Source: CAD feature listing. Evaluate the final solid. Frame: model axes, mm. Give positions to 0.01 mm unless a question says otherwise; leave off trailing zeros. Write each loop counter-clockwise with the first axis right and the second up, starting at its lowest first coordinate (ties: lowest second). Pieces come first, ordered by that corner, then holes. Notation, with made-up numbers: (73, 13.5) -> (112, 13.5) arc R15 cw to (112, 39.5) -> close; hole circle Ø2 at (55, -31). An arc over 180 degrees is marked (long way). Write item = value, one per line.
from build123d import *

# Parameters (mm, degrees)
SKETCH_1_W          = 148.2
SKETCH_1_H          = 100
SKETCH_1_W_2        = 144.2
SKETCH_1_H_2        = 96
EXTRUDE_1_DEPTH     = 4
SKETCH_2_R          = 0.4
CUT_EXTRUDE_1_DEPTH = 125.526342595
SKETCH_3_R          = 0.4
CUT_EXTRUDE_2_DEPTH = 157.458428984


with BuildPart() as part:
    # 草图1 → 凸台-拉伸1 (new body)
    with BuildSketch(Plane(origin=(0, 0, 0), x_dir=(1, 0, 0), z_dir=(0, 1, 0))):
        Rectangle(SKETCH_1_W, SKETCH_1_H)
        Rectangle(SKETCH_1_W_2, SKETCH_1_H_2, mode=Mode.SUBTRACT)
    extrude(amount=EXTRUDE_1_DEPTH)

    # 草图2 → 切除-拉伸1 (cut, through all)
    with BuildSketch(Plane.XY.offset(50)):
        with Locations((0, 2)):
            Circle(SKETCH_2_R)
        with Locations((-60, 2)):
            Circle(SKETCH_2_R)
        with Locations((60, 2)):
            Circle(SKETCH_2_R)
    extrude(amount=-CUT_EXTRUDE_1_DEPTH, mode=Mode.SUBTRACT)

    # 草图3 → 切除-拉伸2 (cut, through all)
    with BuildSketch(Plane.ZY.offset(74.1)):
        with Locations((0, 2)):
            Circle(SKETCH_3_R)
        with Locations((35, 2)):
            Circle(SKETCH_3_R)
        with Locations((-35, 2)):
            Circle(SKETCH_3_R)
    extrude(amount=-CUT_EXTRUDE_2_DEPTH, mode=Mode.SUBTRACT)


solid = part.part
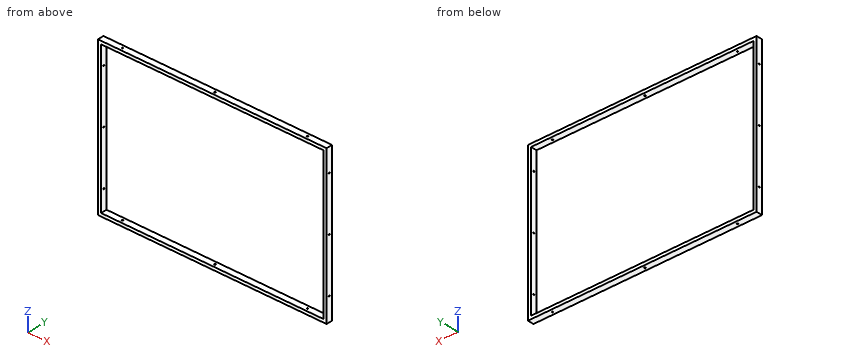
1) Cut plane B-B (z = 25). Return the cut outline in (x, y), then the cut area to 3 significant figures.
Computed:
outline = (-74.1, 0) -> (-72.1, 0) -> (-72.1, 4) -> (-74.1, 4) -> close; (72.1, 0) -> (74.1, 0) -> (74.1, 4) -> (72.1, 4) -> close
area = 16.0 mm²
2) Cut plane C-C (y = 0.6). Return the cut outline in (x, z).
Computed:
outline = (-74.1, -50) -> (74.1, -50) -> (74.1, 50) -> (-74.1, 50) -> close; hole (-72.1, -48) -> (72.1, -48) -> (72.1, 48) -> (-72.1, 48) -> close
3) Material intervals for L1, parallel to Z at x = -43, y = 2.9; L2, parallel to X at y = 3.1, z = -13; L3, parallel to Y at x = 72.8, z = -35, sorted ascending.
Computed:
L1 = -50 to -48, 48 to 50
L2 = -74.1 to -72.1, 72.1 to 74.1
L3 = 0 to 1.6, 2.4 to 4
4) Cut plane A-A (x = 13.5). Return the cut outline in (y, z).
Computed:
outline = (0, -50) -> (4, -50) -> (4, -48) -> (0, -48) -> close; (0, 48) -> (4, 48) -> (4, 50) -> (0, 50) -> close
